```python
from build123d import *

# Parameters (mm, degrees)
BOSS_EXTRUDE1_DEPTH = 69.85
SKETCH2_W           = 50.292
SKETCH2_H           = 12.7
BOSS_EXTRUDE2_DEPTH = 63.5
SKETCH5_R           = 25.146
BOSS_EXTRUDE3_DEPTH = 69.85
SKETCH8_R           = 8.808520998
CUT_EXTRUDE2_DEPTH  = 251.552300113
FILLET7_R           = 12.7


with BuildPart() as part:
    # Sketch1 → Boss-Extrude1 (new body)
    with BuildSketch(Plane.XY):
        Polygon((0, 0), (42.418, 0), (42.418, -35.744914454), (17.018, -35.744914454), (17.018, -74.168), (80.518, -74.168), (80.518, -36.068), (55.118, -36.068), (55.118, 0), (97.536, 0), (97.536, -131.318), (0, -131.318), align=None)
    extrude(amount=BOSS_EXTRUDE1_DEPTH)

    # Sketch2 → Boss-Extrude2 (add)
    with BuildSketch(Plane.XZ.offset(131.318)):
        with Locations((48.768, 6.35)):
            Rectangle(SKETCH2_W, SKETCH2_H)
        with Locations((48.768, 63.5)):
            Rectangle(SKETCH2_W, SKETCH2_H)
    extrude(amount=BOSS_EXTRUDE2_DEPTH)

    # Sketch5 → Boss-Extrude3 (add)
    with BuildSketch(Plane(origin=(0, 0, 0), x_dir=(-1, 0, 0), z_dir=(0, 0, -1))):
        with Locations((-48.768, -194.818)):
            Circle(SKETCH5_R)
    extrude(amount=-BOSS_EXTRUDE3_DEPTH)

    # Sketch8 → Cut-Extrude2 (cut, through all)
    with BuildSketch(Plane.XY.offset(69.85)):
        with Locations((48.768, -194.818)):
            Circle(SKETCH8_R)
    extrude(amount=-CUT_EXTRUDE2_DEPTH, mode=Mode.SUBTRACT)

    # Fillet7
    fillet7_edges = [part.edges().sort_by_distance(p)[0] for p in [
        (21.209, 0, 0),
        (97.536, -65.659, 69.85),
        (76.327, 0, 0),
        (97.536, -65.659, 0),
        (0, -65.659, 0),
        (76.327, 0, 69.85),
        (0, 0, 34.925),
        (97.536, 0, 34.925),
        (97.536, -131.318, 34.925),
        (0, -131.318, 34.925),
        (21.209, 0, 69.85),
        (0, -65.659, 69.85),
    ]]
    fillet(fillet7_edges, radius=FILLET7_R)


solid = part.part
```
CAD build for the part. Positions are in the model's coordinates, mm. A direction names the side the tool comes from. Round coordinates to 2 decimals unless told otherwise and drop trailing zeros. Order: outer loops, then holes, each group sorted by start corner. A loop starts at its lowest first (then second) coordinate and runs counter-clockwise, first axis right, second up. Notation, with made-up numbers: (84, -23.75) -> (96, -23.75) arc R25 ccw to (96, -9.75) -> close; hole circle Ø2 at (-7, 13). An arc over 180 degrees is marked (long way). Write item = value, one per line.
(1) Cut at D-D (y = -104). Write the cut outline in (x, z).
Answers follow:
outline = (0, 12.7) arc R12.7 ccw to (12.7, 0) -> (84.84, 0) arc R12.7 ccw to (97.54, 12.7) -> (97.54, 57.15) arc R12.7 ccw to (84.84, 69.85) -> (12.7, 69.85) arc R12.7 ccw to (0, 57.15) -> close
(2) 3-axis set-ups, long thin cutter, end or side, ignore diameter. For faces 1 (the flat face through (80.518, -55, 34)), 2 (the flat face through (23.622, -163, 63)), 3 (the flat face through (73.914, -163, 63)): which of +Z, -Z, +X, -X, +Y, -Y reach the whole face in a straight line?
Answers follow:
face_1 = +Z, -Z
face_2 = +Z, -Z, -X, -Y
face_3 = +Z, -Z, +X, -Y
(3) Pull direction X, two halves, no side cores. Call faces 4 (the flat face through (23.622, -163, 6)), 5 (the flat face through (68, -36.068, 34)), 6 (the cylindrical face through (70.19, -3.62, 66.03)), 7 (the flat face through (42.418, -18, 34)): +X half, -X half, draft (parallel to the pull), parting line (faces both ways), or undercut.
Answers follow:
face_4 = -X half
face_5 = undercut
face_6 = draft
face_7 = undercut
(4) Drill centre lines: L1, parallel to Z at x = 56.5, y = -164; L2, parallel to Y at x = 69, z = 44; L3, parallel to Y at x = 51, z = 28. Where is each one in solid material? Low to high.
Answers follow:
L1 = 0 to 12.7, 57.15 to 69.85
L2 = -209.75 to -179.89, -131.32 to -74.17, -36.07 to 0
L3 = -219.86 to -203.34, -186.3 to -169.77, -131.32 to -74.17
(5) Cut at A-A (z = 24). Write the cut outline in (x, y), plus the area to 3 significant figures.
Answers follow:
outline = (0, -118.62) arc R12.7 ccw to (12.7, -131.32) -> (84.84, -131.32) arc R12.7 ccw to (97.54, -118.62) -> (97.54, -12.7) arc R12.7 ccw to (84.84, 0) -> (55.12, 0) -> (55.12, -36.07) -> (80.52, -36.07) -> (80.52, -74.17) -> (17.02, -74.17) -> (17.02, -35.74) -> (42.42, -35.74) -> (42.42, 0) -> (12.7, 0) arc R12.7 ccw to (0, -12.7) -> close; circle Ø50.29 at (48.77, -194.82); hole circle Ø17.62 at (48.77, -194.82)
area = 11,500 mm²
(6) Cut at B-B (y = -51). Write the cut outline in (x, z).
Answers follow:
outline = (0, 12.7) arc R12.7 ccw to (12.7, 0) -> (17.02, 0) -> (17.02, 69.85) -> (12.7, 69.85) arc R12.7 ccw to (0, 57.15) -> close; (80.52, 0) -> (84.84, 0) arc R12.7 ccw to (97.54, 12.7) -> (97.54, 57.15) arc R12.7 ccw to (84.84, 69.85) -> (80.52, 69.85) -> close
(7) Cut at C-C (x = 65.5). Write the cut outline in (y, z).
Answers follow:
outline = (-213.59, 0) -> (-74.17, 0) -> (-74.17, 69.85) -> (-213.59, 69.85) -> close; (-36.07, 0) -> (-12.7, 0) arc R12.7 ccw to (0, 12.7) -> (0, 57.15) arc R12.7 ccw to (-12.7, 69.85) -> (-36.07, 69.85) -> close; hole (-176.05, 12.7) -> (-131.32, 12.7) -> (-131.32, 57.15) -> (-176.05, 57.15) -> close
(8) Flat gauge pins, fed straight in: P1, Ø2, axis at x = 32.5, z = 14.5, coming from the -Y side; P2, Ø5, axis at y = -169, z = 39.5, coming from the -X side; P3, Ø6.5, axis at y = -174, z = 65, coming from the -X side; P4, Ø25, axis at x = 50, y = -149.5, coming from the -Z side. Where does each tip first touch, or does it go through?
Answers follow:
P1 = -214.8
P2 = 39.36
P3 = 23.62
P4 = 0
